Source: CAD feature listing. Evaluate the final solid. Frame: model axes, mm. A direction names the side the tool comes from. Give positions to 0.01 mm unless a question says otherwise; leave off trailing zeros. Write each loop counter-clockwise with the first axis right and the second up, starting at its lowest first coordinate (ties: lowest second). Pieces come first, ordered by that corner, then holes. Notation, with made-up numbers: (89, 31) -> (98, 31) arc R22 cw to (98, 59) -> close; hole circle Ø2 at (28.5, 30.5). An arc over 180 degrees is marked (long way). Use one line per item in the form item = value. Start each with the question number.
(1) Cut plane D-D, the plane y = -17. Output: boundary loops of the cut face in (x, z).
(2) Draft query along Y for faces 4 (the face through (0, -4, 5)), 5 (the face through (-3.81, 1.04, 9.29)), 6 (the face through (0, 0, -8)). Return one class per face: pulls with the +Y half, pulls with the -Y half, needs draft (parallel to the pull), parting line crosses it, or undercut.
(3) Cut plane A-A, the plane z = 10.5. Output: boundary loops of the cut face in (x, y) (3 decimals).
(4) Set-up query: faces 1 (the face through (0, 41, -4)), 2 (the face through (-7, -2, 5)), 3 (the face through (-2, -7, 5)). Return all of +Z, -Z, +X, -X, +Y, -Y with unobstructed straight access to the full face (end or side cutting, diameter ignored); none if empty.
(5) Cut plane C-C, the plane z = 1. Output: boundary loops of the cut face in (x, y), and give its area (3 significant figures).
(6) First-contact query: P1, Ø3, axis at y = 0.5, z = -4, coming from the -X side; P2, Ø1.6, axis at y = -41, z = -6, coming from the -X side; P3, Ø1, axis at y = 41, z = -3.5, coming from the +X side. Flat tips, straight axial feed; report the tip coordinate or a pass-through.
(7) Material intervals for line 1 along Y through (x, z) = (0, 10.1); line 2 along X through (y, z) = (6.5, 1); line 3 along X through (y, z) = (6, 8), sorted ascending. Write a range as from..to.
(8) Cut plane B-B, the plane x = 21. Output: boundary loops of the cut face in (y, z), and give its area (3 significant figures).
from build123d import *

# Parameters (mm, degrees)
LEG_SKETCH_R      = 1.15
LEG_DEPTH         = 8
HUB_SKETCH_R      = 8
HUB_SKETCH_R_2    = 1.15
HUB_DEPTH         = 12
CLEARANCE_DEPTH   = 14.5
HUB_CUTOUT_DEPTH  = 5.5
COVER_BOLTS_DEPTH = 12


with BuildPart() as part:
    # Leg-Sketch → Leg (new body)
    with BuildSketch(Plane.XY):
        with BuildLine():
            Line((0, -42), (0, -40))
            ThreePointArc((0, -40), (22.793187837, -20.077432085), (6.099520657, 5.176470588))
            ThreePointArc((6.099520657, 5.176470588), (7.259881704, -3.360672202), (0, -8))
            ThreePointArc((0, -8), (-25, 17), (0, 42))
            Line((0, 42), (0, 40))
            ThreePointArc((0, 40), (-22.793187837, 20.077432085), (-6.099520657, -5.176470588))
            ThreePointArc((-6.099520657, -5.176470588), (-7.259881704, 3.360672202), (0, 8))
            ThreePointArc((0, 8), (25, -17), (0, -42))
        make_face()
        with Locations((0, 6)):
            Circle(LEG_SKETCH_R, mode=Mode.SUBTRACT)
        with Locations((-6, 0)):
            Circle(LEG_SKETCH_R, mode=Mode.SUBTRACT)
        with Locations((0, -6)):
            Circle(LEG_SKETCH_R, mode=Mode.SUBTRACT)
        with Locations((6, 0)):
            Circle(LEG_SKETCH_R, mode=Mode.SUBTRACT)
    extrude(amount=LEG_DEPTH)

    # Hub-Sketch → Hub (add)
    with BuildSketch(Plane(origin=(0, 0, 0), x_dir=(-1, 0, 0), z_dir=(0, 0, -1))):
        Circle(HUB_SKETCH_R)
        with Locations((0, 6)):
            Circle(HUB_SKETCH_R_2, mode=Mode.SUBTRACT)
        with Locations((-6, 0)):
            Circle(HUB_SKETCH_R_2, mode=Mode.SUBTRACT)
        with Locations((0, -6)):
            Circle(HUB_SKETCH_R_2, mode=Mode.SUBTRACT)
        with Locations((6, 0)):
            Circle(HUB_SKETCH_R_2, mode=Mode.SUBTRACT)
    extrude(amount=HUB_DEPTH)

    # Clearance-Sketch → Clearance (cut)
    with BuildSketch(Plane.XY.offset(8)):
        with BuildLine():
            Line((6, 2), (8, 2))
            Line((8, 2), (8, -2))
            Line((8, -2), (6, -2))
            ThreePointArc((6, -2), (4, 0), (6, 2))
        make_face()
        with BuildLine():
            Line((2, -6), (2, -8))
            Line((2, -8), (-2, -8))
            Line((-2, -8), (-2, -6))
            ThreePointArc((-2, -6), (0, -4), (2, -6))
        make_face()
        with BuildLine():
            Line((-6, -2), (-8, -2))
            Line((-8, -2), (-8, 2))
            Line((-8, 2), (-6, 2))
            ThreePointArc((-6, 2), (-4, 0), (-6, -2))
        make_face()
        with BuildLine():
            Line((-2, 6), (-2, 8))
            Line((-2, 8), (2, 8))
            Line((2, 8), (2, 6))
            ThreePointArc((2, 6), (0, 4), (-2, 6))
        make_face()
    extrude(amount=-CLEARANCE_DEPTH, mode=Mode.SUBTRACT)

    # Hub-Cutout-Sketch → Hub-Cutout (cut)
    with BuildSketch(Plane(origin=(0, 0, -12), x_dir=(-1, 0, 0), z_dir=(0, 0, -1))):
        with BuildLine():
            Line((-3.420800345, 1.975), (-6.92820323, 4))
            ThreePointArc((-6.92820323, 4), (2.070552361, -7.72740661), (4, 6.92820323))
            Line((4, 6.92820323), (1.975, 3.420800345))
            ThreePointArc((1.975, 3.420800345), (3.821665179, 0.998686766), (3.396076023, -2.017217799))
            Line((3.396076023, -2.017217799), (4.103182804, -2.72432458))
            Line((4.103182804, -2.72432458), (2.72432458, -4.103182804))
            Line((2.72432458, -4.103182804), (2.017217799, -3.396076023))
            ThreePointArc((2.017217799, -3.396076023), (-2.775720699, -2.810315747), (-3.420800345, 1.975))
        make_face()
    extrude(amount=-HUB_CUTOUT_DEPTH, mode=Mode.SUBTRACT)

    # Cover-Bolts-Sketch → Cover-Bolts (add)
    with BuildSketch(Plane.XY.offset(8)):
        with BuildLine():
            Line((5.656854249, 5.656854249), (0, 0))
            Line((0, 0), (-5.656854249, 5.656854249))
            ThreePointArc((-5.656854249, 5.656854249), (0, -8), (5.656854249, 5.656854249))
        make_face()
    extrude(amount=-COVER_BOLTS_DEPTH)


with BuildPart() as body_2:
    # Mirror 2: mirrored copy
    add(part.part.mirror(Plane.XY))


solid = body_2.part
Geometry says:
q1.outline = (23, -8) -> (25, -8) -> (25, 0) -> (23, 0) -> close
q2.face_4 = pulls with the -Y half
q2.face_5 = undercut
q2.face_6 = needs draft
q3.outline = (-4.103, -2.724) -> (-2.724, -4.103) -> (-2.017, -3.396) arc R3.95 ccw to (3.421, 1.975) -> (6.928, 4) arc R8 ccw to (-4, 6.928) -> (-1.975, 3.421) arc R3.95 ccw to (-3.396, -2.017) -> close; hole circle Ø2.3 at (0, 6)
q4.face_1 = +Z, -Z, +X, +Y
q4.face_2 = +Z, -X
q4.face_3 = +Z, -Y
q5.outline = (-2, 6) -> (-2, 7.75) arc R8 ccw (long way) to (2, 7.75) -> (2, 6) arc R2 cw to start
q5.area = 187 mm^2
q6.P1 = -20
q6.P2 = 0
q6.P3 = 0
q7.line_1 = -3.95..4.85, 7.15..8
q7.line_2 = -4.66..-2, 2..4.66
q7.line_3 = -3.46..-1.15, 1.15..5.29
q8.outline = (-30.56, -8) -> (-26.38, -8) -> (-26.38, 0) -> (-30.56, 0) -> close; (-7.62, -8) -> (-3.44, -8) -> (-3.44, 0) -> (-7.62, 0) -> close
q8.area = 66.9 mm^2
